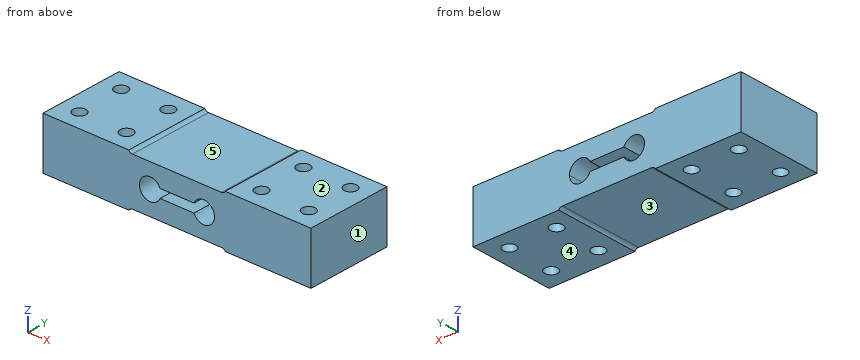
from build123d import *

# Parameters (mm, degrees)
F0_W        = 125
F0_H        = 40
F0_R        = 3
F1_DEPTH    = 24
F3_DEPTH    = 45
F4_W        = 45
F4_H        = 40
F5_DEPTH    = 1
F6_W        = 45
F6_H        = 40
F7_DEPTH    = 1
F8_T1_DEPTH = 40


# Not quite as in the source:
# - a fillet or chamfer that OpenCascade refuses, or shapes differently, is made with other operations: its cross-section is extruded or revolved along the edge and cut away or added


with BuildPart() as f1:
    # F0 (on Top) → F1 (new body)
    with BuildSketch(Plane.XY):
        with Locations((62.5, 20)):
            Rectangle(F0_W, F0_H)
        with Locations((9, 9)):
            Circle(F0_R, mode=Mode.SUBTRACT)
        with Locations((31, 9)):
            Circle(F0_R, mode=Mode.SUBTRACT)
        with Locations((94, 9)):
            Circle(F0_R, mode=Mode.SUBTRACT)
        with Locations((116, 9)):
            Circle(F0_R, mode=Mode.SUBTRACT)
        with Locations((9, 31)):
            Circle(F0_R, mode=Mode.SUBTRACT)
        with Locations((31, 31)):
            Circle(F0_R, mode=Mode.SUBTRACT)
        with Locations((94, 31)):
            Circle(F0_R, mode=Mode.SUBTRACT)
        with Locations((116, 31)):
            Circle(F0_R, mode=Mode.SUBTRACT)
    extrude(amount=F1_DEPTH)

    # F2 (on face) → F3 (cut)
    with BuildSketch(Plane.XZ):
        with BuildLine():
            Line((54, 14), (54.582575695, 14))
            ThreePointArc((54.582575695, 14), (45, 12), (54.582575695, 10))
            Line((54.582575695, 10), (54, 10))
            Line((54, 10), (54, 14))
        make_face()
        with BuildLine():
            ThreePointArc((54.582575695, 10), (54.8945315647, 10.9784517816), (55, 12))
            ThreePointArc((55, 12), (54.8945315647, 13.0215482184), (54.582575695, 14))
            Line((54.582575695, 14), (54, 14))
            Line((54, 14), (54, 10))
            Line((54, 10), (54.582575695, 10))
        make_face()
        with BuildLine():
            ThreePointArc((54.582575695, 14), (54.8945315647, 13.0215482184), (55, 12))
            ThreePointArc((55, 12), (54.8945315647, 10.9784517816), (54.582575695, 10))
            Line((54.582575695, 10), (70.417424305, 10))
            ThreePointArc((70.417424305, 10), (70, 12), (70.417424305, 14))
            Line((70.417424305, 14), (54.582575695, 14))
        make_face()
        with BuildLine():
            Line((71, 14), (70.417424305, 14))
            ThreePointArc((70.417424305, 14), (70, 12), (70.417424305, 10))
            Line((70.417424305, 10), (71, 10))
            Line((71, 10), (71, 14))
        make_face()
        with BuildLine():
            ThreePointArc((80, 12), (76.0215482184, 16.8945315647), (70.417424305, 14))
            Line((70.417424305, 14), (71, 14))
            Line((71, 14), (71, 10))
            Line((71, 10), (70.417424305, 10))
            ThreePointArc((70.417424305, 10), (76.0215482184, 7.1054684353), (80, 12))
        make_face()
    extrude(amount=-F3_DEPTH, mode=Mode.SUBTRACT)

    # F4 (on face) → F5 (cut)
    with BuildSketch(Plane.XY.offset(24)):
        with Locations((62.5, 20)):
            Rectangle(F4_W, F4_H)
    extrude(amount=-F5_DEPTH, mode=Mode.SUBTRACT)

    # F6 (on face) → F7 (cut)
    with BuildSketch(Plane(origin=(0, 0, 0), x_dir=(1, 0, 0), z_dir=(0, 0, -1))):
        with Locations((62.5, -20)):
            Rectangle(F6_W, F6_H)
    extrude(amount=-F7_DEPTH, mode=Mode.SUBTRACT)

    # F8: fillet of radius 2 on 4 edges, made by hand

    # F8_s2 → F8_t1 (join)
    with BuildSketch(Plane.XZ.offset(-40)):
        with BuildLine():
            ThreePointArc((41.7320508076, 1), (40.7320508076, 0.7320508076), (40, 0))
            Line((40, 0), (40, 1))
            Line((40, 1), (41.7320508076, 1))
        make_face()
        with BuildLine():
            ThreePointArc((85, 0), (84.2679491924, 0.7320508076), (83.2679491924, 1))
            Line((83.2679491924, 1), (85, 1))
            Line((85, 1), (85, 0))
        make_face()
        with BuildLine():
            ThreePointArc((83.2679491924, 23), (84.2679491924, 23.2679491924), (85, 24))
            Line((85, 24), (85, 23))
            Line((85, 23), (83.2679491924, 23))
        make_face()
        with BuildLine():
            ThreePointArc((40, 24), (40.7320508076, 23.2679491924), (41.7320508076, 23))
            Line((41.7320508076, 23), (40, 23))
            Line((40, 23), (40, 24))
        make_face()
    extrude(amount=F8_T1_DEPTH)


solid = f1.part
Geometry: final body of the model. Coordinates: model frame, mm. Face numbers are marked on the shaded views. A direction names the side the tool comes from. Give positions to 0.01 mm unless a question says otherwise; leave off trailing zeros. Loops run counter-clockwise (first coordinate to the right, second up) from the corner with the lowest first, then second, coordinate; pieces in that order, holes last. Notation, with made-up numbers: M 40.25,-14.5 L 62.25,-14.5 A25 ccw 62.25,1.5 Z; hole C 11.25,48 d6. An arc over 180 degrees is marked long. Put each result on its own line as item: value.
1) Material intervals for L1, parallel to Y at x = 116, z = 14.5; L2, parallel to Y at x = 28.5, z = 9.25; L3, parallel to X at y = 17, z = 8.5, sorted ascending. Write a range as from..to.
Computed values:
L1: y = 0..6, 12..28, 34..40
L2: y = 0..7.34, 10.66..29.34, 32.66..40
L3: x = 0..46.43, 53.57..71.43, 78.57..125
2) Mould query, pull axis X, two halves, no side actions, for the marked faces 1, 2 and 3. Classes: released by +X, released by -X, zero draft, split by the parting line, or undercut.
Computed values:
face 1: released by +X
face 2: zero draft
face 3: undercut
3) Reachability of the marked faces 4 and 5 from +Z, -Z, +X, -X, +Y, -Y: full face, straight path, thin tool, end or side. Return the list, or none.
Computed values:
face 4: -Z, +X, -X, +Y, -Y
face 5: +Z, +Y, -Y
4) Cut plane B-B, the plane x = 31. Return the cut outline in (y, z), plus the area to 3 significant figures.
Computed values:
outline: M 0,0 L 6,0 L 6,24 L 0,24 Z; M 12,0 L 28,0 L 28,24 L 12,24 Z; M 34,0 L 40,0 L 40,24 L 34,24 Z
area: 672 mm^2
5) Cut plane A-A, the plane y = 9. Give the number of separate pieces and of enclosed holes in the cut face, plus the area to 3 significant figures.
Computed values:
separate pieces: 5
enclosed holes: 1
area: 2,120 mm^2
6) Cut plane D-D, the plane y = 4. Return the cut outline in (x, z).
Computed values:
outline: M 0,0 L 40,0 A2 cw 41.73,1 L 83.27,1 A2 cw 85,0 L 125,0 L 125,24 L 85,24 A2 cw 83.27,23 L 41.73,23 A2 cw 40,24 L 0,24 Z; hole M 54.58,10 L 70.42,10 A5 ccw long 70.42,14 L 54.58,14 A5 ccw long Z
7) First-contact query: P1, Ø5, axis at x = 53.5, y = 5.5, coming from the +Z side; P2, Ø8, axis at x = 61.5, y = 20.5, coming from the -Z side. Flat tips, straight axial feed; report the tip coordinate or a pass-through.
Computed values:
P1: stops at z = 23
P2: stops at z = 1
